Here's how the part is built. I have some questions about the finished solid (model axes, mm). Give positions to 0.01 mm unless a question says otherwise; leave off trailing zeros. Write each loop counter-clockwise with the first axis right and the second up, starting at its lowest first coordinate (ties: lowest second). Pieces come first, ordered by that corner, then holes. Notation, with made-up numbers: (6, -18.75) - (48, -18.75) arc R25 ccw to (48, 17.25) - close; hole circle Ø6 at (-19.75, 46.5). An arc over 180 degrees is marked (long way). One line per item, written item: value. Start each with the question number.
1) Imagine slicing it at A-A on y = 18. Write out the boundary of the cut face in (x, z).
2) Imagine slicing it at C-C on z = -8. Write out the boundary of the cut face in (x, y).
3) Imagine slicing it at B-B on x = 0. Write out the boundary of the cut face in (y, z).
4) Please list where these lines run through material, in increasing order: L1, parallel to X at y = 9, z = -13; L2, parallel to X at y = -2, z = -5.5; L3, parallel to Y at x = 7, z = -2.5. Write a range as [from, to].
5) I'm going to push flat-ended pins straight in: P1, Ø4, axis at y = 2.5, z = -7.5, coming from the -X side; P2, Ø1.5, axis at x = 11, z = 13, coming from the -Y side; P3, Ø2, axis at x = 4.5, z = 9, coming from the -Y side. Where does each tip first touch, or does it pass through?
from build123d import *

# Parameters (mm, degrees)
EXTRUDE_1_DEPTH = 20


with BuildPart() as part:
    # 草图1 → 凸台-拉伸1 (new, symmetric)
    with BuildSketch(Plane.XY):
        with BuildLine():
            Line((47.577439338, 13.227810722), (45.99529172, -21.662716293))
            Line((45.99529172, -21.662716293), (15.689460366, -21.662716293))
            Line((15.689460366, -21.662716293), (-5.318631208, -8.468303377))
            ThreePointArc((-5.318631208, -8.468303377), (-8.583413456, 5.130790723), (4.940460041, 8.694357629))
            ThreePointArc((4.940460041, 8.694357629), (18.534857961, 7.551984283), (28.214467512, 17.165403581))
            ThreePointArc((28.214467512, 17.165403581), (39.580485947, 23.480235483), (47.577439338, 13.227810722))
        make_face()
    extrude(amount=EXTRUDE_1_DEPTH, both=True)


solid = part.part
Numbers:
1. outline: (28.57, -20) - (46.61, -20) - (46.61, 20) - (28.57, 20) - close
2. outline: (-5.32, -8.47) - (15.69, -21.66) - (46, -21.66) - (47.58, 13.23) arc R10 ccw to (28.21, 17.17) arc R16.26 cw to (4.94, 8.69) arc R10 ccw to start
3. outline: (-11.81, -20) - (10, -20) - (10, 20) - (-11.81, 20) - close
4. L1: [-4.36, 4.36], [21.52, 47.39]
4. L2: [-9.8, 46.89]
4. L3: [-16.21, 7.71]
5. P1: x = -9.99
5. P2: y = -19.19
5. P3: y = -15.26
